For this review, take the finished solid that the model builds, in its own axes (mm). Face numbers are marked on the shaded views. A direction names the side the tool comes from. Give positions to 0.01 mm unless a question says otherwise; leave off trailing zeros. Order: outer loops, then holes, each group sorted by start corner. A loop starts at its lowest first (then second) coordinate and runs counter-clockwise, first axis right, second up. Notation, with made-up numbers: (20, 61) - (55, 61) arc R28 cw to (55, 83) - close; hole circle Ø6 at (63.25, 69). An arc over 180 degrees is marked (long way). Use a Markdown table: item, result. Add a question column.
1) Mouldability with a two-part tool opening along X and no side actions: class the marked faces 4, 5, 6 and 7 as released by +X, released by -X, zero draft, split by the parting line, or undercut.
2) We need section D-D on z = -30.5. Write out the cut boundary in (x, y), then the cut area to 3 significant figures.
3) We need section A-A on y = 0.5. Write out the cut boundary in (x, z).
4) We need section B-B on x = -7. Write out the cut boundary in (y, z), then the cut area to 3 significant figures.
5) Clearance check with flat-ended pins moving along their axes: P1, Ø1.5, axis at y = 24.5, z = -23.5, coming from the +X side; P2, Ø5, axis at x = 8.5, y = 9, coming from the -Z side; P3, Ø5, axis at x = -14.5, z = -11, coming from the +Y side; P4, Ø3, axis at x = 18.5, z = -16.5, coming from the -Y side. State where each tip first meets the part, or that it passes through.
6) We need section C-C on y = 12.25. Write out the cut boundary in (x, z).
7) Machinability: for the marked faces 1, 2 and 3, which of the approach directions +Z, -Z, +X, -X, +Y, -Y give a long, thin tool a straight path to every point of the face, cutting with its end or side? Answer none if there is none.
8) Wall thickness on L1, parallel to Y at x = 3.5, z = -30.5; L2, parallel to X at y = 5.5, z = -6.5; L3, parallel to X at y = 18.5, z = -13.5: over which ranges is each line inside the solid? List them lowest first.
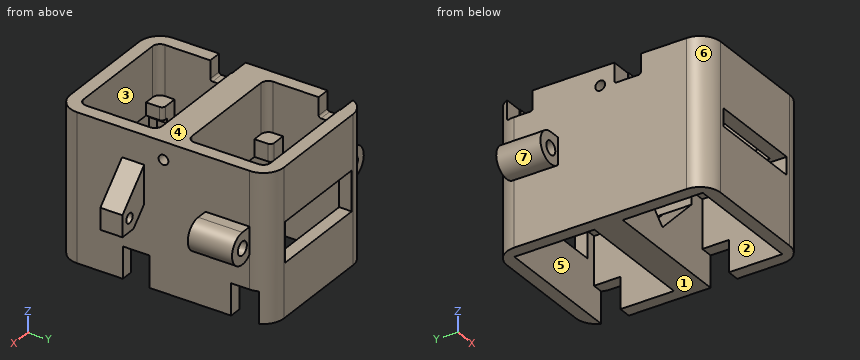
```python
from build123d import *

# Parameters (mm, degrees)
EXTRUDE_2_DEPTH      = 11.22
EXTRUDE_3_DEPTH      = 3.88
CUT_EXTRUDE_1_DEPTH  = 4.65
SKETCH_8_R           = 3.525
SKETCH_8_R_2         = 1.525
EXTRUDE_5_DEPTH      = 10
SKETCH_9_W           = 22.64
SKETCH_9_H           = 3
CUT_EXTRUDE_3_DEPTH  = 3
SKETCH_10_W          = 21.46
SKETCH_10_H          = 6.88
CUT_EXTRUDE_4_DEPTH  = 1
SKETCH_11_R          = 1.1
EXTRUDE_6_DEPTH      = 5
SKETCH_12_R          = 1.1
CUT_EXTRUDE_5_DEPTH  = 8
CUT_EXTRUDE_START    = -8
SKETCH_13_R          = 1.1
CUT_EXTRUDE_6_DEPTH  = 8
SKETCH_14_W          = 6.52
SKETCH_14_H          = 9.58
EXTRUDE_7_DEPTH      = 3
SKETCH_15_W          = 27.1
SKETCH_15_H          = 42.6
EXTRUDE_8_DEPTH      = 18
SKETCH_16_W          = 27.1
SKETCH_16_H          = 6.4
EXTRUDE_9_DEPTH      = 15
CUT_EXTRUDE_8_REACH  = 51.09
CUT_EXTRUDE_9_REACH  = 62.949
SKETCH_18_W          = 7.1
SKETCH_18_H          = 6
CUT_EXTRUDE_START_2  = -2.85
SKETCH_19_W          = 21.46
SKETCH_19_H          = 1
SKETCH_19_H_2        = 3
CUT_EXTRUDE_10_DEPTH = 2.85
CUT_EXTRUDE_11_REACH = 65.204
SKETCH_20_W          = 22.64
SKETCH_20_H          = 6


with BuildPart() as part:
    # 草图2 → 凸台-拉伸2 (new body)
    with BuildSketch(Plane.XY):
        with BuildLine():
            ThreePointArc((-16.4, -7.25), (-15.038046533, -10.538046533), (-11.75, -11.9))
            Line((-11.75, -11.9), (11.75, -11.9))
            ThreePointArc((11.75, -11.9), (15.038046533, -10.538046533), (16.4, -7.25))
            Line((16.4, -7.25), (16.4, 31.75))
            ThreePointArc((16.4, 31.75), (15.038046533, 35.038046533), (11.75, 36.4))
            Line((11.75, 36.4), (-11.75, 36.4))
            ThreePointArc((-11.75, 36.4), (-15.038046533, 35.038046533), (-16.4, 31.75))
            Line((-16.4, 31.75), (-16.4, -7.25))
        make_face()
        with BuildLine():
            Line((13.4, 7.25), (13.4, -7.25))
            ThreePointArc((13.4, -7.25), (12.916726189, -8.416726189), (11.75, -8.9))
            Line((11.75, -8.9), (-11.75, -8.9))
            ThreePointArc((-11.75, -8.9), (-12.916726189, -8.416726189), (-13.4, -7.25))
            Line((-13.4, -7.25), (-13.4, 7.25))
            ThreePointArc((-13.4, 7.25), (-12.916726189, 8.416726189), (-11.75, 8.9))
            Line((-11.75, 8.9), (11.75, 8.9))
            ThreePointArc((11.75, 8.9), (12.916726189, 8.416726189), (13.4, 7.25))
        make_face(mode=Mode.SUBTRACT)
        with BuildLine():
            Line((-11.75, 33.4), (11.75, 33.4))
            ThreePointArc((11.75, 33.4), (12.916726189, 32.916726189), (13.4, 31.75))
            Line((13.4, 31.75), (13.4, 17.25))
            ThreePointArc((13.4, 17.25), (12.916726189, 16.083273811), (11.75, 15.6))
            Line((11.75, 15.6), (-11.75, 15.6))
            ThreePointArc((-11.75, 15.6), (-12.916726189, 16.083273811), (-13.4, 17.25))
            Line((-13.4, 17.25), (-13.4, 31.75))
            ThreePointArc((-13.4, 31.75), (-12.916726189, 32.916726189), (-11.75, 33.4))
        make_face(mode=Mode.SUBTRACT)
    extrude(amount=-EXTRUDE_2_DEPTH)

    # 草图3 → 凸台-拉伸3 (add)
    with BuildSketch(Plane(origin=(0, 0, -11.22), x_dir=(-1, 0, 0), z_dir=(0, 0, -1))):
        with BuildLine():
            ThreePointArc((11.75, -11.9), (15.038046533, -10.538046533), (16.4, -7.25))
            Line((16.4, -7.25), (16.4, 31.75))
            ThreePointArc((16.4, 31.75), (15.038046533, 35.038046533), (11.75, 36.4))
            Line((11.75, 36.4), (-11.75, 36.4))
            ThreePointArc((-11.75, 36.4), (-15.038046533, 35.038046533), (-16.4, 31.75))
            Line((-16.4, 31.75), (-16.4, -7.25))
            ThreePointArc((-16.4, -7.25), (-15.038046533, -10.538046533), (-11.75, -11.9))
            Line((-11.75, -11.9), (11.75, -11.9))
        make_face()
        with BuildLine():
            Line((13.4, -5.02), (10.37, -5.02))
            ThreePointArc((10.37, -5.02), (9.768959236, -5.268959236), (9.52, -5.87))
            Line((9.52, -5.87), (9.52, -8.9))
            Line((9.52, -8.9), (-9.52, -8.9))
            Line((-9.52, -8.9), (-9.52, -5.87))
            ThreePointArc((-9.52, -5.87), (-9.768959236, -5.268959236), (-10.37, -5.02))
            Line((-10.37, -5.02), (-13.4, -5.02))
            Line((-13.4, -5.02), (-13.4, 6.82))
            Line((-13.4, 6.82), (-11.67, 6.82))
            ThreePointArc((-11.67, 6.82), (-11.422512627, 6.922512627), (-11.32, 7.17))
            Line((-11.32, 7.17), (-11.32, 8.9))
            Line((-11.32, 8.9), (11.32, 8.9))
            Line((11.32, 8.9), (11.32, 7.17))
            ThreePointArc((11.32, 7.17), (11.422512627, 6.922512627), (11.67, 6.82))
            Line((11.67, 6.82), (13.4, 6.82))
            Line((13.4, 6.82), (13.4, -5.02))
        make_face(mode=Mode.SUBTRACT)
        with BuildLine():
            Line((13.4, 31.32), (13.4, 19.48))
            Line((13.4, 19.48), (10.37, 19.48))
            ThreePointArc((10.37, 19.48), (9.768959236, 19.231040764), (9.52, 18.63))
            Line((9.52, 18.63), (9.52, 15.6))
            Line((9.52, 15.6), (-9.52, 15.6))
            Line((-9.52, 15.6), (-9.52, 18.63))
            ThreePointArc((-9.52, 18.63), (-9.768959236, 19.231040764), (-10.37, 19.48))
            Line((-10.37, 19.48), (-13.4, 19.48))
            Line((-13.4, 19.48), (-13.4, 31.32))
            Line((-13.4, 31.32), (-11.67, 31.32))
            ThreePointArc((-11.67, 31.32), (-11.422512627, 31.422512627), (-11.32, 31.67))
            Line((-11.32, 31.67), (-11.32, 33.4))
            Line((-11.32, 33.4), (11.32, 33.4))
            Line((11.32, 33.4), (11.32, 31.67))
            ThreePointArc((11.32, 31.67), (11.422512627, 31.422512627), (11.67, 31.32))
            Line((11.67, 31.32), (13.4, 31.32))
        make_face(mode=Mode.SUBTRACT)
    extrude(amount=EXTRUDE_3_DEPTH)

    # 草图4 → 切除-拉伸1 (cut)
    with BuildSketch(Plane.ZY.offset(16.4)):
        with BuildLine():
            Line((0.3, 9.05), (-4, 9.05))
            ThreePointArc((-4, 9.05), (-4.353553391, 8.903553391), (-4.5, 8.55))
            Line((-4.5, 8.55), (-4.5, 3.55))
            ThreePointArc((-4.5, 3.55), (-4.353553391, 3.196446609), (-4, 3.05))
            Line((-4, 3.05), (0.3, 3.05))
            Line((0.3, 3.05), (0.3, 9.05))
        make_face()
        with BuildLine():
            Line((0.3, 33.55), (-4, 33.55))
            ThreePointArc((-4, 33.55), (-4.353553391, 33.403553391), (-4.5, 33.05))
            Line((-4.5, 33.05), (-4.5, 28.05))
            ThreePointArc((-4.5, 28.05), (-4.353553391, 27.696446609), (-4, 27.55))
            Line((-4, 27.55), (0.3, 27.55))
            Line((0.3, 27.55), (0.3, 33.55))
        make_face()
    extrude(amount=-CUT_EXTRUDE_1_DEPTH, mode=Mode.SUBTRACT)

    # 草图8 → 凸台-拉伸5 (add)
    # profile 1 of 2: a face of its own
    with BuildSketch(Plane(origin=(0, 31.75, 0), x_dir=(1, 0, 0), z_dir=(0, 1, 0))):
        with Locations((18.9, 15.755)):
            Circle(SKETCH_8_R)
        with Locations(Location((18.9, 15.755, 0), (0, 0, 270))):
            Circle(SKETCH_8_R_2, mode=Mode.SUBTRACT)
    # profile 2 of 2: a face of its own
    with BuildSketch(Plane(origin=(0, 31.75, 0), x_dir=(1, 0, 0), z_dir=(0, 1, 0))):
        with BuildLine():
            Line((15.375, 12.23), (18.9, 12.23))
            ThreePointArc((18.9, 12.23), (16.407448596, 13.262448596), (15.375, 15.755))
            Line((15.375, 15.755), (15.375, 12.23))
        make_face()
    extrude_5 = extrude(amount=-EXTRUDE_5_DEPTH)

    # 镜向1: 凸台-拉伸5 across plane
    add(extrude_5.mirror(Plane(origin=(0, 0, 0), x_dir=(0, 0, 1), z_dir=(1, 0, 0))))

    # 草图9 → 切除-拉伸3 (cut)
    with BuildSketch(Plane(origin=(0, 0, -15.1), x_dir=(-1, 0, 0), z_dir=(0, 0, -1))):
        with Locations((0, 34.9)):
            Rectangle(SKETCH_9_W, SKETCH_9_H)
    extrude(amount=-CUT_EXTRUDE_3_DEPTH, mode=Mode.SUBTRACT)

    # 草图10 → 切除-拉伸4 (cut)
    with BuildSketch(Plane(origin=(0, 0, -15.1), x_dir=(-1, 0, 0), z_dir=(0, 0, -1))):
        with Locations((0, -8.46)):
            Rectangle(SKETCH_10_W, SKETCH_10_H)
    extrude(amount=-CUT_EXTRUDE_4_DEPTH, mode=Mode.SUBTRACT)

    # 草图11 → 凸台-拉伸6 (add)
    with BuildSketch(Plane(origin=(0, 2.890336251, 0), x_dir=(1, 0, 0), z_dir=(0, 1, 0))):
        Polygon((23.795757056, 13.912359313), (23.795757056, 18.755), (20.055, 18.755), (16.4, 15.1), (16.4, 6.516602257), align=None)
        with Locations(Location((21.395757056, 15.755, 0), (0, 0, 180))):
            Circle(SKETCH_11_R, mode=Mode.SUBTRACT)
    extrude(amount=EXTRUDE_6_DEPTH)

    # 草图12 → 切除-拉伸5 (cut)
    with BuildSketch(Plane.ZY.offset(16.4)):
        with Locations((-4, 12.25)):
            Circle(SKETCH_12_R)
    extrude(amount=-CUT_EXTRUDE_5_DEPTH, mode=Mode.SUBTRACT)

    # 草图13 → 切除-拉伸6 (cut)
    with BuildSketch(Plane(origin=(16.4, 0, 0), x_dir=(0, 0, -1), z_dir=(1, 0, 0)).offset(CUT_EXTRUDE_START)):
        with Locations(Location((4, 12.25, 0), (0, 0, 180))):
            Circle(SKETCH_13_R)
    extrude(amount=CUT_EXTRUDE_6_DEPTH, mode=Mode.SUBTRACT)

    # 草图14 → 凸台-拉伸7 (add)
    with BuildSketch(Plane(origin=(0, 0, -15.1), x_dir=(-1, 0, 0), z_dir=(0, 0, -1))):
        with Locations((-13.14, 13.84)):
            Rectangle(SKETCH_14_W, SKETCH_14_H)
        with Locations((13.14, 13.84)):
            Rectangle(SKETCH_14_W, SKETCH_14_H)
    extrude(amount=EXTRUDE_7_DEPTH)

    # 草图15 → 凸台-拉伸8 (add)
    with BuildSketch(Plane(origin=(0, 0, -15.1), x_dir=(-1, 0, 0), z_dir=(0, 0, -1))):
        with BuildLine():
            Line((16.4, 9.05), (16.4, 18.63))
            Line((16.4, 18.63), (16.4, 31.75))
            ThreePointArc((16.4, 31.75), (15.038046533, 35.038046533), (11.75, 36.4))
            Line((11.75, 36.4), (-11.75, 36.4))
            ThreePointArc((-11.75, 36.4), (-15.038046533, 35.038046533), (-16.4, 31.75))
            Line((-16.4, 31.75), (-16.4, 21.75))
            Line((-16.4, 21.75), (-16.4, 18.63))
            Line((-16.4, 18.63), (-16.4, 9.05))
            Line((-16.4, 9.05), (-16.4, 2.890336251))
            Line((-16.4, 2.890336251), (-16.4, -7.25))
            ThreePointArc((-16.4, -7.25), (-15.038046533, -10.538046533), (-11.75, -11.9))
            Line((-11.75, -11.9), (11.75, -11.9))
            ThreePointArc((11.75, -11.9), (15.038046533, -10.538046533), (16.4, -7.25))
            Line((16.4, -7.25), (16.4, 9.05))
        make_face()
        with Locations((0, 12.25)):
            Rectangle(SKETCH_15_W, SKETCH_15_H, mode=Mode.SUBTRACT)
    extrude(amount=EXTRUDE_8_DEPTH)

    # 草图16 → 凸台-拉伸9 (add)
    with BuildSketch(Plane(origin=(0, 0, -18.1), x_dir=(-1, 0, 0), z_dir=(0, 0, -1))):
        with Locations((0, 12.25)):
            Rectangle(SKETCH_16_W, SKETCH_16_H)
    extrude(amount=EXTRUDE_9_DEPTH)

    # 草图17 → 切除-拉伸8 (cut, up to next)
    with BuildSketch(Plane.XZ.offset(-9.05), mode=Mode.PRIVATE) as cut_extrude_8_sk1:
        Polygon((-9.88, -18.1), (0, -27.98), (9.88, -18.1), align=None)
    cut_extrude_8_tool1 = extrude(cut_extrude_8_sk1.sketch, amount=-CUT_EXTRUDE_8_REACH, mode=Mode.PRIVATE) & part.part
    add(cut_extrude_8_tool1.solids().sort_by_distance((0, 9.05, -21.393333))[0], mode=Mode.SUBTRACT)

    # 草图18 → 切除-拉伸9 (cut, up to next)
    with BuildSketch(Plane.ZY.offset(-13.55), mode=Mode.PRIVATE) as cut_extrude_9_sk1:
        with Locations((-29.55, 6.05)):
            Rectangle(SKETCH_18_W, SKETCH_18_H)
    cut_extrude_9_tool1 = extrude(cut_extrude_9_sk1.sketch, amount=-CUT_EXTRUDE_9_REACH, mode=Mode.PRIVATE) & part.part
    # 草图18 → 切除-拉伸9 (cut, up to next)
    with BuildSketch(Plane.ZY.offset(-13.55), mode=Mode.PRIVATE) as cut_extrude_9_sk2:
        with Locations((-29.55, 30.55)):
            Rectangle(SKETCH_18_W, SKETCH_18_H)
    cut_extrude_9_tool2 = extrude(cut_extrude_9_sk2.sketch, amount=-CUT_EXTRUDE_9_REACH, mode=Mode.PRIVATE) & part.part
    add(cut_extrude_9_tool1.solids().sort_by_distance((13.55, 6.05, -29.55))[0], mode=Mode.SUBTRACT)
    add(cut_extrude_9_tool2.solids().sort_by_distance((13.55, 30.55, -29.55))[0], mode=Mode.SUBTRACT)

    # 草图19 → 切除-拉伸10 (cut)
    with BuildSketch(Plane.XZ.offset(11.9).offset(CUT_EXTRUDE_START_2)):
        with Locations((0, -14.6)):
            Rectangle(SKETCH_19_W, SKETCH_19_H)
        with Locations((0, -16.6)):
            Rectangle(SKETCH_19_W, SKETCH_19_H_2)
    extrude(amount=CUT_EXTRUDE_10_DEPTH, mode=Mode.SUBTRACT)

    # 草图20 → 切除-拉伸11 (cut, up to next)
    with BuildSketch(Plane(origin=(0, 36.4, 0), x_dir=(1, 0, 0), z_dir=(0, 1, 0)), mode=Mode.PRIVATE) as cut_extrude_11_sk1:
        with Locations((0, 18.1)):
            Rectangle(SKETCH_20_W, SKETCH_20_H)
    cut_extrude_11_tool1 = extrude(cut_extrude_11_sk1.sketch, amount=-CUT_EXTRUDE_11_REACH, mode=Mode.PRIVATE) & part.part
    add(cut_extrude_11_tool1.solids().sort_by_distance((0, 36.4, -18.1))[0], mode=Mode.SUBTRACT)


solid = part.part
```
Checked values:
| question | item | result |
|---|---|---|
| 1 | face 4 | zero draft |
| 1 | face 5 | undercut |
| 1 | face 6 | released by -X |
| 1 | face 7 | undercut |
| 2 | outline | (-16.4, -7.25) arc R4.65 ccw to (-11.75, -11.9) - (11.75, -11.9) arc R4.65 ccw to (16.4, -7.25) - (16.4, 3.05) - (13.55, 3.05) - (13.55, -9.05) - (-13.55, -9.05) - (-13.55, 9.05) - (16.4, 9.05) - (16.4, 27.55) - (13.55, 27.55) - (13.55, 15.45) - (-13.55, 15.45) - (-13.55, 33.55) - (16.04, 33.55) arc R4.65 ccw to (11.75, 36.4) - (-11.75, 36.4) arc R4.65 ccw to (-16.4, 31.75) - close |
| 2 | area | 551 mm² |
| 3 | outline | (-16.4, -33.1) - (-13.55, -33.1) - (-13.55, -15.1) - (-13.4, -15.1) - (-13.4, 0) - (-16.4, 0) - close; (13.4, -15.1) - (13.55, -15.1) - (13.55, -33.1) - (16.4, -33.1) - (16.4, 0) - (13.4, 0) - close |
| 4 | outline | (-11.9, -33.1) - (-9.05, -33.1) - (-9.05, -18.1) - (-11.9, -18.1) - close; (-11.9, -14.1) - (-8.9, -14.1) - (-8.9, 0) - (-11.9, 0) - close; (8.9, -15.1) - (15.6, -15.1) - (15.6, 0) - (8.9, 0) - close; (9.05, -33.1) - (15.45, -33.1) - (15.45, -20.98) - (9.05, -20.98) - close; (33.4, -12.1) - (36.4, -12.1) - (36.4, 0) - (33.4, 0) - close; (33.55, -33.1) - (36.4, -33.1) - (36.4, -21.1) - (33.55, -21.1) - close |
| 4 | area | 334 mm² |
| 5 | P1 | x = 16.4 |
| 5 | P2 | z = -33.1 |
| 5 | P3 | y = 36.39 |
| 5 | P4 | y = 2.89 |
| 6 | outline | (-16.4, -33.1) - (16.4, -33.1) - (16.4, -5.1) - (8.4, -5.1) - (8.4, -2.9) - (16.4, -2.9) - (16.4, 0) - (-16.4, 0) - (-16.4, -2.9) - (-8.4, -2.9) - (-8.4, -5.1) - (-16.4, -5.1) - close; hole (-9.88, -18.1) - (0, -27.98) - (9.88, -18.1) - (9.88, -15.1) - (-9.88, -15.1) - close |
| 7 | face 1 | -Z, +X, -X, +Y, -Y |
| 7 | face 2 | -Z |
| 7 | face 3 | +Z |
| 8 | L1 | -11.9 to -9.05, 9.05 to 15.45, 33.55 to 36.4 |
| 8 | L2 | -16.4 to -13.4, 13.4 to 16.4 |
| 8 | L3 | -16.4 to -9.52, 9.52 to 16.4 |
